Source: CAD feature listing. Evaluate the final solid. Frame: model axes, mm. Face numbers are marked on the shaded views. A direction names the side the tool comes from. Give positions to 0.01 mm unless a question says otherwise; leave off trailing zeros. Write each loop counter-clockwise with the first axis right and the second up, starting at its lowest first coordinate (ties: lowest second). Pieces come first, ordered by that corner, then holes.
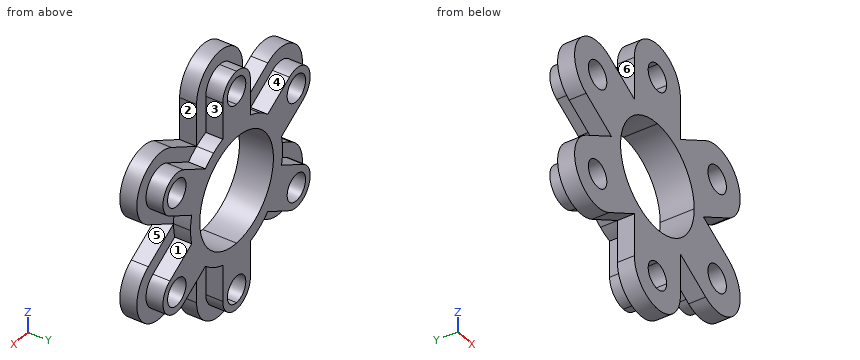
```python
from build123d import *

# Parameters (mm, degrees)
SKETCH1_R           = 4
BOSS_EXTRUDE1_DEPTH = 10
BOSS_EXTRUDE2_DEPTH = 5


with BuildPart() as part:
    # Sketch1 → Boss-Extrude1 (new body)
    # profile 1 of 2: a face of its own
    with BuildSketch(Plane(origin=(0, 0, 0), x_dir=(1, 0, 0), z_dir=(0, 1, 0))):
        with BuildLine():
            Line((0, -34), (0, -36))
            ThreePointArc((0, -36), (4.242640687, -34.242640687), (6, -30))
            Line((6, -30), (6, -19.078784028))
            ThreePointArc((6, -19.078784028), (8.048160261, -18.309208514), (10, -17.320508076))
            ThreePointArc((10, -17.320508076), (11.832159566, -16.124515497), (13.522711642, -14.735544437))
            Line((13.522711642, -14.735544437), (22.980762114, -20.196152423))
            ThreePointArc((22.980762114, -20.196152423), (31.176914536, -18), (28.980762114, -9.803847577))
            Line((28.980762114, -9.803847577), (19.522711642, -4.343239591))
            ThreePointArc((19.522711642, -4.343239591), (19.880319827, -2.184693018), (20, 0))
            ThreePointArc((20, 0), (19.880319827, 2.184693018), (19.522711642, 4.343239591))
            Line((19.522711642, 4.343239591), (28.980762114, 9.803847577))
            ThreePointArc((28.980762114, 9.803847577), (31.176914536, 18), (22.980762114, 20.196152423))
            Line((22.980762114, 20.196152423), (13.522711642, 14.735544437))
            ThreePointArc((13.522711642, 14.735544437), (11.832159566, 16.124515497), (10, 17.320508076))
            ThreePointArc((10, 17.320508076), (8.048160261, 18.309208514), (6, 19.078784028))
            Line((6, 19.078784028), (6, 30))
            ThreePointArc((6, 30), (4.242640687, 34.242640687), (0, 36))
            Line((0, 36), (0, 34))
            ThreePointArc((0, 34), (2.828427125, 32.828427125), (4, 30))
            ThreePointArc((4, 30), (2.828427125, 27.171572875), (0, 26))
            Line((0, 26), (0, 16))
            ThreePointArc((0, 16), (11.313708499, 11.313708499), (16, 0))
            ThreePointArc((16, 0), (11.313708499, -11.313708499), (0, -16))
            Line((0, -16), (0, -26))
            ThreePointArc((0, -26), (2.828427125, -27.171572875), (4, -30))
            ThreePointArc((4, -30), (2.828427125, -32.828427125), (0, -34))
        make_face()
        with Locations(Location((25.980762114, -15, 0), (0, 0, 270))):
            Circle(SKETCH1_R, mode=Mode.SUBTRACT)
        with Locations(Location((25.980762114, 15, 0), (0, 0, 270))):
            Circle(SKETCH1_R, mode=Mode.SUBTRACT)
    # profile 2 of 2: a face of its own
    with BuildSketch(Plane(origin=(0, 0, 0), x_dir=(1, 0, 0), z_dir=(0, 1, 0))):
        with BuildLine():
            ThreePointArc((-6, -30), (-4.242640687, -34.242640687), (0, -36))
            Line((0, -36), (0, -34))
            ThreePointArc((0, -34), (-4, -30), (0, -26))
            Line((0, -26), (0, -16))
            ThreePointArc((0, -16), (-16, 0), (0, 16))
            Line((0, 16), (0, 26))
            ThreePointArc((0, 26), (-4, 30), (0, 34))
            Line((0, 34), (0, 36))
            ThreePointArc((0, 36), (-4.242640687, 34.242640687), (-6, 30))
            Line((-6, 30), (-6, 19.078784028))
            ThreePointArc((-6, 19.078784028), (-8.048160261, 18.309208514), (-10, 17.320508076))
            ThreePointArc((-10, 17.320508076), (-11.832159566, 16.124515497), (-13.522711642, 14.735544437))
            Line((-13.522711642, 14.735544437), (-22.980762114, 20.196152423))
            ThreePointArc((-22.980762114, 20.196152423), (-31.176914536, 18), (-28.980762114, 9.803847577))
            Line((-28.980762114, 9.803847577), (-19.522711642, 4.343239591))
            ThreePointArc((-19.522711642, 4.343239591), (-19.880319827, 2.184693018), (-20, 0))
            ThreePointArc((-20, 0), (-19.880319827, -2.184693018), (-19.522711642, -4.343239591))
            Line((-19.522711642, -4.343239591), (-28.980762114, -9.803847577))
            ThreePointArc((-28.980762114, -9.803847577), (-31.176914536, -18), (-22.980762114, -20.196152423))
            Line((-22.980762114, -20.196152423), (-13.522711642, -14.735544437))
            ThreePointArc((-13.522711642, -14.735544437), (-11.832159566, -16.124515497), (-10, -17.320508076))
            ThreePointArc((-10, -17.320508076), (-8.048160261, -18.309208514), (-6, -19.078784028))
            Line((-6, -19.078784028), (-6, -30))
        make_face()
        with Locations(Location((-25.980762114, -15, 0), (0, 0, 270))):
            Circle(SKETCH1_R, mode=Mode.SUBTRACT)
        with Locations(Location((-25.980762114, 15, 0), (0, 0, 270))):
            Circle(SKETCH1_R, mode=Mode.SUBTRACT)
    extrude(amount=BOSS_EXTRUDE1_DEPTH)

    # Sketch1_5 → Boss-Extrude2 (add)
    with BuildSketch(Plane(origin=(0, 0, 0), x_dir=(1, 0, 0), z_dir=(0, 1, 0))):
        with BuildLine():
            ThreePointArc((-20, 0), (-19.880319827, -2.184693018), (-19.522711642, -4.343239591))
            Line((-19.522711642, -4.343239591), (-28.980762114, -9.803847577))
            ThreePointArc((-28.980762114, -9.803847577), (-31.176914536, -18), (-22.980762114, -20.196152423))
            Line((-22.980762114, -20.196152423), (-13.522711642, -14.735544437))
            ThreePointArc((-13.522711642, -14.735544437), (-11.832159566, -16.124515497), (-10, -17.320508076))
            Line((-10, -17.320508076), (-20.980762114, -23.660254038))
            ThreePointArc((-20.980762114, -23.660254038), (-34.641016151, -20), (-30.980762114, -6.339745962))
            Line((-30.980762114, -6.339745962), (-20, 0))
        make_face()
        with BuildLine():
            ThreePointArc((20, 0), (19.880319827, 2.184693018), (19.522711642, 4.343239591))
            Line((19.522711642, 4.343239591), (28.980762114, 9.803847577))
            ThreePointArc((28.980762114, 9.803847577), (31.176914536, 18), (22.980762114, 20.196152423))
            Line((22.980762114, 20.196152423), (13.522711642, 14.735544437))
            ThreePointArc((13.522711642, 14.735544437), (11.832159566, 16.124515497), (10, 17.320508076))
            Line((10, 17.320508076), (20.980762114, 23.660254038))
            ThreePointArc((20.980762114, 23.660254038), (34.641016151, 20), (30.980762114, 6.339745962))
            Line((30.980762114, 6.339745962), (20, 0))
        make_face()
        with BuildLine():
            ThreePointArc((10, -17.320508076), (11.832159566, -16.124515497), (13.522711642, -14.735544437))
            Line((13.522711642, -14.735544437), (22.980762114, -20.196152423))
            ThreePointArc((22.980762114, -20.196152423), (31.176914536, -18), (28.980762114, -9.803847577))
            Line((28.980762114, -9.803847577), (19.522711642, -4.343239591))
            ThreePointArc((19.522711642, -4.343239591), (19.880319827, -2.184693018), (20, 0))
            Line((20, 0), (30.980762114, -6.339745962))
            ThreePointArc((30.980762114, -6.339745962), (34.641016151, -20), (20.980762114, -23.660254038))
            Line((20.980762114, -23.660254038), (10, -17.320508076))
        make_face()
        with BuildLine():
            ThreePointArc((-6, -30), (0, -36), (6, -30))
            Line((6, -30), (6, -19.078784028))
            ThreePointArc((6, -19.078784028), (8.048160261, -18.309208514), (10, -17.320508076))
            Line((10, -17.320508076), (10, -30))
            ThreePointArc((10, -30), (0, -40), (-10, -30))
            Line((-10, -30), (-10, -17.320508076))
            ThreePointArc((-10, -17.320508076), (-8.048160261, -18.309208514), (-6, -19.078784028))
            Line((-6, -19.078784028), (-6, -30))
        make_face()
        with BuildLine():
            ThreePointArc((10, 30), (0, 40), (-10, 30))
            Line((-10, 30), (-10, 17.320508076))
            ThreePointArc((-10, 17.320508076), (-8.048160261, 18.309208514), (-6, 19.078784028))
            Line((-6, 19.078784028), (-6, 30))
            ThreePointArc((-6, 30), (0, 36), (6, 30))
            Line((6, 30), (6, 19.078784028))
            ThreePointArc((6, 19.078784028), (8.048160261, 18.309208514), (10, 17.320508076))
            Line((10, 17.320508076), (10, 30))
        make_face()
        with BuildLine():
            ThreePointArc((-20.980762114, 23.660254038), (-34.641016151, 20), (-30.980762114, 6.339745962))
            Line((-30.980762114, 6.339745962), (-20, 0))
            ThreePointArc((-20, 0), (-19.880319827, 2.184693018), (-19.522711642, 4.343239591))
            Line((-19.522711642, 4.343239591), (-28.980762114, 9.803847577))
            ThreePointArc((-28.980762114, 9.803847577), (-31.176914536, 18), (-22.980762114, 20.196152423))
            Line((-22.980762114, 20.196152423), (-13.522711642, 14.735544437))
            ThreePointArc((-13.522711642, 14.735544437), (-11.832159566, 16.124515497), (-10, 17.320508076))
            Line((-10, 17.320508076), (-20.980762114, 23.660254038))
        make_face()
    extrude(amount=BOSS_EXTRUDE2_DEPTH)


solid = part.part
```
1. Section query A-A (y = 3). Return loops of the section in (x, z), plus the area to 3 significant figures.
2. Access query for the marked faces 1, 2 and 3. Directions: +Z, -Z, +X, -X, +Y, -Y. A direction counts if a zero-diameter tool reaches every point of the face in a straight line with its end or side. Return the directions, or none.
3. Section query B-B (y = 7). Give the number of separate pieces and of enclosed holes in the cut face, plus the area to 3 significant figures.
4. Pin query (flat end, axial travel): P1, Ø1.5, axis at x = 4.5, y = 5.5, coming from the -Z side; P2, Ø5, axis at x = -25.98, z = -15, coming from the +Y side; P3, Ø10.5, axis at x = -25.98, z = 15, coming from the -Y side; P4, Ø1.5, axis at y = 3.5, z = 30, coming from the -X side. Return the tip coordinate at first contact, or that it passes through.
5. Pull-direction query (Z, two-part tool) for the marked faces 4, 5 and 6; classes: pulls with the +Z half, pulls with the -Z half, needs draft (parallel to the pull), parting line crosses it, or undercut.
6. Line query: probe 1 along Z at (x, y) = (29, 7.25) (3 decimals); probe 2 along Z at (x, y) = (28, 8); probe 3 along X at (y, z) = (4, -16.5). Output: solid intervals per line, ascending.
The answers:
1. outline: (-30.98, -6.34) arc R10 ccw to (-20.98, -23.66) - (-10, -17.32) - (-10, -30) arc R10 ccw to (10, -30) - (10, -17.32) - (20.98, -23.66) arc R10 ccw to (30.98, -6.34) - (20, 0) - (30.98, 6.34) arc R10 ccw to (20.98, 23.66) - (10, 17.32) - (10, 30) arc R10 ccw to (-10, 30) - (-10, 17.32) - (-20.98, 23.66) arc R10 ccw to (-30.98, 6.34) - (-20, 0) - close; hole circle Ø8 at (-25.98, -15); hole circle Ø8 at (-25.98, 15); hole circle Ø32 at (0, 0); hole circle Ø8 at (0, -30); hole circle Ø8 at (0, 30); hole circle Ø8 at (25.98, -15); hole circle Ø8 at (25.98, 15)
1. area: 2,400 mm2
2. face 1: +X, +Y
2. face 2: +Z, +Y, -Y
2. face 3: +Z, +Y
3. separate pieces: 1
3. enclosed holes: 7
3. area: 1,230 mm2
4. P1: stops at z = -39.19
4. P2: passes through
4. P3: stops at y = 0
4. P4: stops at x = -10
5. face 4: pulls with the +Z half
5. face 5: undercut
5. face 6: needs draft
6. probe 1: z = -20.185 to -17.624, -12.376 to -9.815, 9.815 to 12.376, 17.624 to 20.185
6. probe 2: z = -20.65 to -18.45, -11.55 to -9.24, 9.24 to 11.55, 18.45 to 20.65
6. probe 3: x = -35.87 to -29.69, -22.27 to 22.27, 29.69 to 35.87
